Read the model definition and answer for the solid it produces. Units are mm, in the model's axes. A direction names the side the tool comes from. Coordinates: 2 decimals unless noted, no trailing zeros. Write each loop counter-clockwise with the first axis right and the second up, starting at its lowest first coordinate (ties: lowest second). Pieces come first, ordered by that corner, then holes.
1) Find the intervals of material crossed by line 1 (Y direction, x = 0.5, z = -12.7); line 2 (Y direction, x = 12.7, z = -23.9); line 3 (X direction, y = 14.5, z = -2.75), in increasing order.
2) Determine the mould class of faces 1 (the face through (13, 16, -22.86)), 2 (the face through (24, 0, -13)), 3 (the face through (12.16, 16.62, -24.11)) for opening direction Y: +Y half, -Y half, draft (parallel to the pull), parting line (faces both ways), or undercut.
3) Which of the six approach directions +Z, -Z, +X, -X, +Y, -Y give full straight-line access (tool end or side, diameter ignored) to faces 4 (the face through (13, 16, -2.54)), 5 (the face through (13, 16, 0))?
4) The part is cut by section D-D (x = 12.7). Determine the outline of the cut face in (y, z), then the cut area to 3 significant figures.
5) Each of these flat-tipped pins is pushed along its axis until it touches: pin 1 Ø10 at (x, z) = (3.5, -13) entering from -Y; pin 2 Ø6 at (x, z) = (19, -7) entering from +Y. Where does it stop, or does it pass through?
6) The part is cut by section C-C (x = 16.5). Determine the outline of the cut face in (y, z), then the cut area to 3 significant figures.
7) The part is cut by section B-B (y = 6.35). Determine the outline of the cut face in (x, z).
8) The part is cut by section A-A (z = -17.75). Determine the outline of the cut face in (x, y), then the cut area to 3 significant figures.
from build123d import *

# Parameters (mm, degrees)
SKETCH1_W           = 25.4
SKETCH1_H           = 25.4
SKETCH1_W_2         = 20.32
SKETCH1_H_2         = 20.32
EXTRUDE_THIN1_DEPTH = 31.75
SKETCH2_R           = 2.4892
CUT_EXTRUDE1_DEPTH  = 26.4
SKETCH3_R           = 2.4892
CUT_EXTRUDE2_DEPTH  = 26.4


with BuildPart() as part:
    # Sketch1 → Extrude-Thin1 (new body)
    with BuildSketch(Plane(origin=(0, 0, 0), x_dir=(1, 0, 0), z_dir=(0, 1, 0))):
        with Locations((12.7, 12.7)):
            Rectangle(SKETCH1_W, SKETCH1_H)
        with Locations((12.7, 12.7)):
            Rectangle(SKETCH1_W_2, SKETCH1_H_2, mode=Mode.SUBTRACT)
    extrude(amount=EXTRUDE_THIN1_DEPTH)

    # Sketch2 → Cut-Extrude1 (cut, through all)
    with BuildSketch(Plane.XY):
        with Locations((12.7, 19.05)):
            Circle(SKETCH2_R)
        with Locations((12.7, 6.35)):
            Circle(SKETCH2_R)
    extrude(amount=-CUT_EXTRUDE1_DEPTH, mode=Mode.SUBTRACT)

    # Sketch3 → Cut-Extrude2 (cut, through all)
    with BuildSketch(Plane.ZY):
        with Locations((-12.7, 25.4)):
            Circle(SKETCH3_R)
        with Locations((-12.7, 12.7)):
            Circle(SKETCH3_R)
    extrude(amount=-CUT_EXTRUDE2_DEPTH, mode=Mode.SUBTRACT)


solid = part.part
Reported:
1. line 1: y = 0 to 10.21, 15.19 to 22.91, 27.89 to 31.75
1. line 2: y = 0 to 3.86, 8.84 to 16.56, 21.54 to 31.75
1. line 3: x = 0 to 2.54, 22.86 to 25.4
2. face 1: draft
2. face 2: -Y half
2. face 3: undercut
3. face 4: +Y, -Y
3. face 5: +Z, +X, -X, +Y, -Y
4. outline: (0, -25.4) - (3.86, -25.4) - (3.86, -22.86) - (0, -22.86) - close; (0, -2.54) - (3.86, -2.54) - (3.86, 0) - (0, 0) - close; (8.84, -25.4) - (16.56, -25.4) - (16.56, -22.86) - (8.84, -22.86) - close; (8.84, -2.54) - (16.56, -2.54) - (16.56, 0) - (8.84, 0) - close; (21.54, -25.4) - (31.75, -25.4) - (31.75, -22.86) - (21.54, -22.86) - close; (21.54, -2.54) - (31.75, -2.54) - (31.75, 0) - (21.54, 0) - close
4. area: 111 mm2
5. pin 1: stops at y = 0
5. pin 2: passes through
6. outline: (0, -25.4) - (31.75, -25.4) - (31.75, -22.86) - (0, -22.86) - close; (0, -2.54) - (31.75, -2.54) - (31.75, 0) - (0, 0) - close
6. area: 161 mm2
7. outline: (0, -25.4) - (10.21, -25.4) - (10.21, -22.86) - (2.54, -22.86) - (2.54, -2.54) - (10.21, -2.54) - (10.21, 0) - (0, 0) - close; (15.19, -25.4) - (25.4, -25.4) - (25.4, 0) - (15.19, 0) - (15.19, -2.54) - (22.86, -2.54) - (22.86, -22.86) - (15.19, -22.86) - close
8. outline: (0, 0) - (2.54, 0) - (2.54, 31.75) - (0, 31.75) - close; (22.86, 0) - (25.4, 0) - (25.4, 31.75) - (22.86, 31.75) - close
8. area: 161 mm2
